Read the model definition and answer for the solid it produces. Units are mm, in the model's axes. Face numbers are marked on the shaded views. A direction names the side the tool comes from. Round coordinates to 2 decimals unless told otherwise and drop trailing zeros. Order: outer loops, then holes, each group sorted by start corner. A loop starts at its lowest first (then second) coordinate and runs counter-clockwise, first axis right, second up. Notation, with made-up numbers: (-19.5, 78) -> (36.5, 78) arc R12 cw to (36.5, 84) -> close; hole circle Ø3 at (12.25, 76.25). An arc over 180 degrees is marked (long way). Answer as a JSON object with one key per item and string values. Group by question number.
Item 1: Consider probe 1 along X at (y, z) = (-9.5, 6); probe 2 along Z at (x, y) = (-13.5, -9.35); probe 3 along X at (y, z) = (-2.25, 3.5). Determine where each line is inside the solid, lowest interval first. Write a range as from..to.
Item 2: Section A-A, the plane x = 5.5 is taken. Write down the section's boundary in (y, z).
Item 3: Section C-C, the plane x = -13.5 is taken. Write down the section's boundary in (y, z).
Item 4: Given P1, Ø5, axis at x = -4.5, z = 10, coming from the -Y side; P2, Ø3, axis at y = -13, z = 5, coming from the +X side; P3, Ø4, axis at x = -14, z = 7, coming from the -Y side, each flat-ended and moving along its own axis, determine where each tip first touches the part or whether it passes through.
Item 5: Section B-B, the plane z = 1.75 is taken. Write down the section's boundary in (x, y).
Item 6: For the marked faces 1, 2 and 3, determine the directions among +Z, -Z, +X, -X, +Y, -Y from which every point of the face is accessible in a straight line to the end or side of a thin tool.
Item 7: Section D-D, the plane y = 5.75 is taken. Write down the section's boundary in (x, z).
from build123d import *

# Parameters (mm, degrees)
SALIENTE_EXTRUIR1_DEPTH = 12
CROQUIS2_OUTSIDE_W      = 42.878
CROQUIS2_OUTSIDE_H      = 22.878
CROQUIS2_OUTSIDE_R      = 5.5
CORTAR_EXTRUIR1_DEPTH   = 6.285514833
CROQUIS3_OUTSIDE_W      = 42.878
CROQUIS3_OUTSIDE_H      = 22.878
CROQUIS3_OUTSIDE_R      = 2.5
CORTAR_EXTRUIR2_DEPTH   = 2.285514833
CROQUIS4_R              = 1
CORTAR_EXTRUIR3_DEPTH   = 12


with BuildPart() as part:
    # Croquis1 → Saliente-Extruir1 (new body)
    with BuildSketch(Plane.XY):
        Polygon((-16, -7.537010796), (-11, -7.5), (-11, 7.5), (11, 7.5), (11, -7.5), (16, -7.537010796), (16, -10.537010796), (11, -10.537010796), (11, -14.537010796), (11, -18.537010796), (8, -18.537010796), (8, -20.822525629), (3, -20.822525629), (3, -18.537010796), (0, -18.537010796), (0, -14.537010796), (-11, -14.537010796), (-11, -10.537010796), (-16, -10.537010796), align=None)
    extrude(amount=SALIENTE_EXTRUIR1_DEPTH)

    # Croquis2 outside → Cortar-Extruir1 (cut)
    with BuildSketch(Plane.XZ.offset(20.822525629)):
        with Locations((0, 6)):
            Rectangle(CROQUIS2_OUTSIDE_W, CROQUIS2_OUTSIDE_H)
        with Locations(Location((5.5, 6, 0), (0, 0, 297.035691789))):
            Circle(CROQUIS2_OUTSIDE_R, mode=Mode.SUBTRACT)
    extrude(amount=-CORTAR_EXTRUIR1_DEPTH, mode=Mode.SUBTRACT)

    # Croquis3 outside → Cortar-Extruir2 (cut)
    with BuildSketch(Plane.XZ.offset(20.822525629)):
        with Locations((0, 6)):
            Rectangle(CROQUIS3_OUTSIDE_W, CROQUIS3_OUTSIDE_H)
        with Locations(Location((5.5, 6, 0), (0, 0, 270))):
            Circle(CROQUIS3_OUTSIDE_R, mode=Mode.SUBTRACT)
    extrude(amount=-CORTAR_EXTRUIR2_DEPTH, mode=Mode.SUBTRACT)

    # Croquis4 → Cortar-Extruir3 (cut)
    with BuildSketch(Plane.XZ.offset(10.537010796)):
        with Locations((-13.5, 6)):
            Circle(CROQUIS4_R)
        with Locations((13.5, 6)):
            Circle(CROQUIS4_R)
    extrude(amount=-CORTAR_EXTRUIR3_DEPTH, mode=Mode.SUBTRACT)


solid = part.part
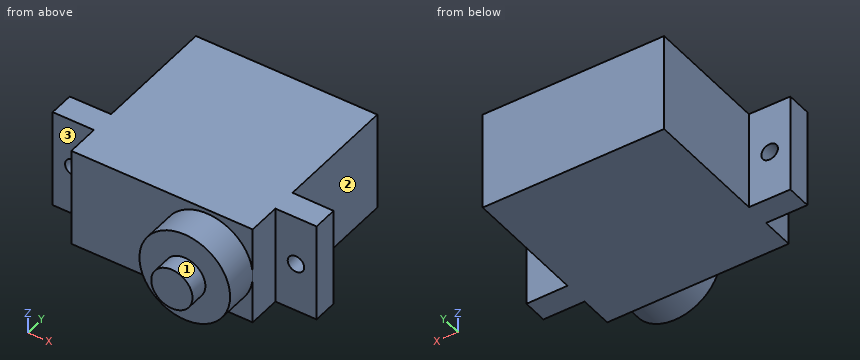
Values found:
{
 "1": {"probe 1": "-16..-14.5, -12.5..12.5, 14.5..16", "probe 2": "0..5, 7..12", "probe 3": "-11..11"},
 "2": {"outline": "(-20.82, 3.5) -> (-18.54, 3.5) -> (-18.54, 0.5) -> (-14.54, 0.5) -> (-14.54, 0) -> (7.5, 0) -> (7.5, 12) -> (-14.54, 12) -> (-14.54, 11.5) -> (-18.54, 11.5) -> (-18.54, 8.5) -> (-20.82, 8.5) -> close"},
 "3": {"outline": "(-10.54, 0) -> (-7.52, 0) -> (-7.52, 5) -> (-10.54, 5) -> close; (-10.54, 7) -> (-7.52, 7) -> (-7.52, 12) -> (-10.54, 12) -> close"},
 "4": {"P1": "y = -14.54", "P2": "x = 11", "P3": "y = -10.54"},
 "5": {"outline": "(-16, -10.54) -> (-11, -10.54) -> (-11, -14.54) -> (2.01, -14.54) -> (2.01, -18.54) -> (8.99, -18.54) -> (8.99, -14.54) -> (11, -14.54) -> (11, -10.54) -> (16, -10.54) -> (16, -7.54) -> (11, -7.5) -> (11, 7.5) -> (-11, 7.5) -> (-11, -7.5) -> (-16, -7.54) -> close"},
 "6": {"face 1": "-Y", "face 2": "+Z, -Z, +X, +Y", "face 3": "+Z, -Z, -X, -Y"},
 "7": {"outline": "(-11, 0) -> (11, 0) -> (11, 12) -> (-11, 12) -> close"}
}
